For this review, take the finished solid that the model builds, in its own axes (mm). Coordinates: 2 decimals unless noted, no trailing zeros. Order: outer loops, then holes, each group sorted by start corner. A loop starts at its lowest first (then second) coordinate and runs counter-clockwise, first axis right, second up. Notation, with made-up numbers: (49.5, -11.5) - (81.5, -11.5) arc R22 ccw to (81.5, 8.5) - close; hole circle Ø7 at (-39.5, 55.25). An arc over 180 degrees is marked (long way). One line per item, written item: value. Start each with the question number.
(1) Clearance check with a flat-ended pin moving along its axis: pin 1 (5 mm diameter, centred on x = -97, y = -5, fed in from -Z). State where the tip first meets the part, or that it passes through.
(2) Consider section A-A on z = 0.8. Count the separate pieces of the cut face and the enclosed holes in it, then the cut area to 3 significant figures.
(3) To check wall thickness, follow line 1 along X through (y, z) = (72.5, 1.8); line 2 along Y through (x, z) = (98, 0.6). State the ranges of each line that lie inside material, in increasing order.
(4) Consider section B-B on x = 132. Write out the cut boundary in (y, z).
```python
from build123d import *

# Parameters (mm, degrees)
F0_W     = 478
F0_H     = 195
F1_DEPTH = 5
F2_D     = 8.25
F3_D     = 10.3


with BuildPart() as f1:
    # F0 (on Top) → F1 (new body)
    with BuildSketch(Plane.XY):
        Rectangle(F0_W, F0_H)
    extrude(amount=F1_DEPTH)

    # F2 (through all)
    with Locations(Plane(origin=(0, 0, 0), x_dir=(1, 0, 0), z_dir=(0, 0, -1))):
        with Locations((-229, -56), (-229, 5), (-229, 66), (-167, -56), (-167, 5), (-167, 66), (-97, 66), (-97, 5), (-97, -56), (-35, -56), (-35, 5), (-35, 66), (35, 66), (35, 5), (35, -56), (97, -56), (97, 5), (97, 66), (167, 66), (167, 5), (167, -56), (229, -56), (229, 5), (229, 66)):
            Hole(F2_D / 2)

    # F3 (through all)
    with Locations(Plane(origin=(0, 0, 0), x_dir=(1, 0, 0), z_dir=(0, 0, -1))):
        with Locations((-132, -72.5), (-132, 67.5), (0, -72.5), (0, 67.5), (132, -72.5), (132, 67.5)):
            Hole(F3_D / 2)


solid = f1.part
```
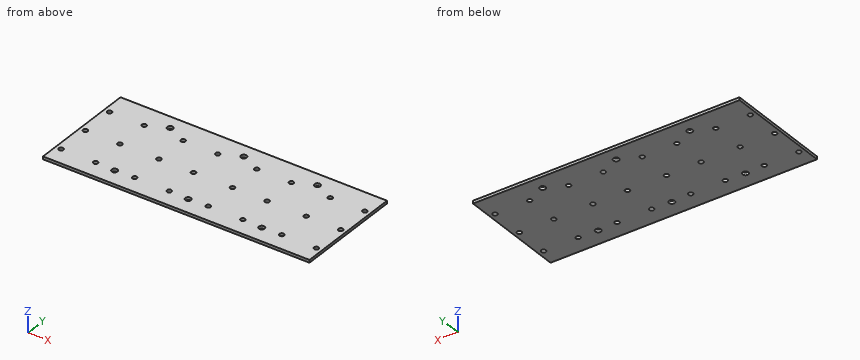
Geometry check:
1. pin 1: passes through
2. separate pieces: 1
2. enclosed holes: 30
2. area: 91,400 mm^2
3. line 1: x = -239 to -137.15, -126.85 to -5.15, 5.15 to 126.85, 137.15 to 239
3. line 2: y = -97.5 to -70, -62 to -9, -1 to 52, 60 to 97.5
4. outline: (-97.5, 0) - (-72.65, 0) - (-72.65, 5) - (-97.5, 5) - close; (-62.35, 0) - (67.35, 0) - (67.35, 5) - (-62.35, 5) - close; (77.65, 0) - (97.5, 0) - (97.5, 5) - (77.65, 5) - close
